Could you check a few things on this model? Use its own coordinates, in mm. Face numbers are marked on the shaded views. A direction names the side the tool comes from. Coordinates: 2 decimals unless noted, no trailing zeros. Order: outer loops, then holes, each group sorted by start corner. A loop starts at its lowest first (then second) coordinate and runs counter-clockwise, first axis right, second up. Notation, with made-up numbers: (-28, 32) - (-22, 32) arc R30 ccw to (-22, 68) - close; hole circle Ø5 at (2.25, -28). An arc over 180 degrees is marked (long way). One line per item, written item: value.
from build123d import *

# Parameters (mm, degrees)
BOSS_EXTRU_2_DEPTH = 6


with BuildPart() as part:
    # Esquisse1 → Boss.-Extru.2 (new body)
    with BuildSketch(Plane.XY):
        with BuildLine():
            Line((-16, 0), (16, 0))
            Line((16, 0), (16, 16))
            Line((16, 16), (12.051970793, 21))
            ThreePointArc((12.051970793, 21), (0, 17.5), (-12.051970793, 21))
            Line((-12.051970793, 21), (-16, 16))
            Line((-16, 16), (-16, 0))
        make_face()
        with BuildLine():
            Line((-7, 13), (7, 13))
            ThreePointArc((7, 13), (12, 8), (7, 3))
            Line((7, 3), (-7, 3))
            ThreePointArc((-7, 3), (-12, 8), (-7, 13))
        make_face(mode=Mode.SUBTRACT)
    extrude(amount=-BOSS_EXTRU_2_DEPTH)


solid = part.part
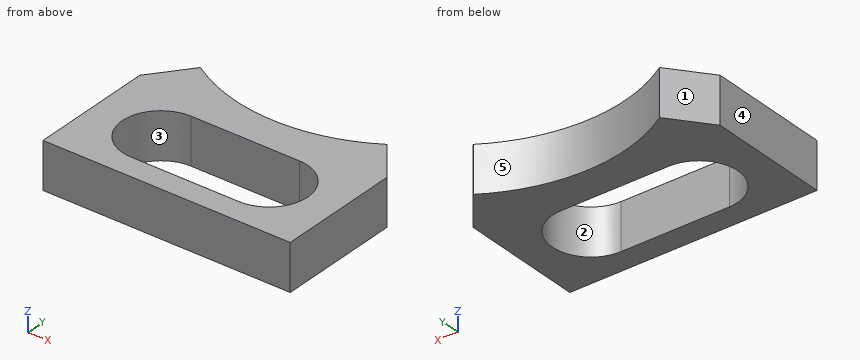
Item 1: For the marked faces 1 and 2, which set-ups out of +Z, -Z, +X, -X, +Y, -Y let a thin tool reach every point of the face, with its end or its side?
Conclusion:
face 1: +Z, -Z, -X, +Y
face 2: +Z, -Z
Item 2: I'm going to push flat-ended pins straight in: pin 1 Ø1.5 at (x, z) = (5.5, -4.5) entering from -Y; pin 2 Ø1.8 at (x, z) = (-3, -1.5) entering from +Y. Where does each tip first touch, or does it pass through?
Conclusion:
pin 1: y = 0
pin 2: y = 17.84
Item 3: I want a section at B-B on z = -5.5. Please give me the cut outline in (x, y), then the cut area to 3 significant figures.
Conclusion:
outline: (-16, 0) - (16, 0) - (16, 16) - (12.05, 21) arc R22.5 cw to (-12.05, 21) - (-16, 16) - close; hole (-7, 3) - (7, 3) arc R5 ccw to (7, 13) - (-7, 13) arc R5 ccw to start
area: 377 mm²
Item 4: I want a section at D-D on x = -14. Please give me the cut outline in (y, z).
Conclusion:
outline: (0, -6) - (18.53, -6) - (18.53, 0) - (0, 0) - close
Item 5: I want a section at A-A on y = 8. Please give me the cut outline in (x, z), then the cut area to 3 significant figures.
Conclusion:
outline: (-16, -6) - (-12, -6) - (-12, 0) - (-16, 0) - close; (12, -6) - (16, -6) - (16, 0) - (12, 0) - close
area: 48.0 mm²
Item 6: I want a section at C-C on x = 0.5. Please give me the cut outline in (y, z), then the cut area to 3 significant figures.
Conclusion:
outline: (0, -6) - (3, -6) - (3, 0) - (0, 0) - close; (13, -6) - (17.51, -6) - (17.51, 0) - (13, 0) - close
area: 45.0 mm²
Item 7: Thinking about a two-plate mould opening in Y: for the marked faces 3, 4 and 5, which applies, pulls with the +Y half, pulls with the -Y half, needs draft (parallel to the pull), parting line crosses it, or undercut?
Conclusion:
face 3: undercut
face 4: needs draft
face 5: pulls with the +Y half
Item 8: If I drill on probe 1 along X at (y, z) = (7.75, -2.3); probe 2 along Y at (x, z) = (3.5, -3.75); probe 3 along Y at (x, z) = (-8, -4.35), over which ranges is the centre line in solid material (lowest first)?
Conclusion:
probe 1: -16 to -11.99, 11.99 to 16
probe 2: 0 to 3, 13 to 17.77
probe 3: 0 to 3.1, 12.9 to 18.97
